from build123d import *

# Parameters (mm, degrees)
F0_R     = 5
F0_W     = 15
F0_H     = 20
F1_DEPTH = 1.6
F2_R     = 1
F3_DEPTH = 25


with BuildPart() as f1:
    # F0 (on Front) → F1 (new body)
    with BuildSketch(Plane.XZ):
        Polygon((28, 71), (-24.5, 71), (-24.5, 30), (-28, 30), (-28, -102), (8, -102), (8, -82), (28, -82), align=None)
        with Locations((-14.37, -78.52)):
            Circle(F0_R, mode=Mode.SUBTRACT)
        with Locations((-14.37, -55.02)):
            Circle(F0_R, mode=Mode.SUBTRACT)
        with Locations((-14.58, -35.06)):
            Rectangle(F0_W, F0_H, mode=Mode.SUBTRACT)
        Polygon((1.52, -25.06), (9.02, -25.06), (16.52, -25.06), (16.52, -45.06), (9.02, -45.06), (1.52, -45.06), align=None, mode=Mode.SUBTRACT)
    extrude(amount=-F1_DEPTH)

    # F2 (on face) → F3 (cut)
    with BuildSketch(Plane.XZ):
        with Locations((0, 25.5)):
            Circle(F2_R)
        with Locations((0, 68)):
            Circle(F2_R)
        with Locations((23, 17)):
            Circle(F2_R)
        with Locations((23, -17)):
            Circle(F2_R)
        with Locations((-23, -10)):
            Circle(F2_R)
        with Locations((0, -58)):
            Circle(F2_R)
        with Locations((-5, -78.5)):
            Circle(F2_R)
    extrude(amount=-F3_DEPTH, mode=Mode.SUBTRACT)


solid = f1.part
Could you check a few things on this model? Use its own coordinates, in mm. Give positions to 0.01 mm unless a question says otherwise; leave off trailing zeros. Order: outer loops, then holes, each group sorted by start corner. A loop starts at its lowest first (then second) coordinate and runs counter-clockwise, first axis right, second up.
Item 1: If we section it at B-B, the plane y = 0.8: Count the separate pieces of the cut face and the enclosed holes in it, plus the area to 3 significant figures.
Item 2: If we section it at C-C, the plane z = 54: Write out the boundary of the cut face in (x, y), plus the area to 3 significant figures.
Item 3: I'm going to push flat-ended pins straight in: pin 1 (0.5 mm diameter, centred on y = 1, z = 56.5, fed in from -X); pin 2 (1.8 mm diameter, centred on x = -5, z = -78.5, fed in from +Y); pin 3 (13 mm diameter, centred on x = -14.37, z = -78.52, fed in from -Y). Where does each tip first touch, or does it pass through?
Item 4: If we mould it in two halves opening along X, with no side actions, what happens to faces 1 (the face through (0, 0, -14)), 2 (the face through (-9.6, 0.79, -53.52))? For each: pulls with the +X half, pulls with the -X half, needs draft (parallel to the pull), parting line crosses it, or undercut.
Item 5: If we section it at A-A, the plane x = -12: Write out the boundary of the cut face in (y, z), plus the area to 3 significant figures.
Item 6: I need wall thicknesses on line 1 (Z direction, x = 0, y = 1); line 2 (X direction, y = 1.3, z = -43.5); line 3 (X direction, y = 0.6, z = -78.5). Which ranges of each line are inside material? Lowest first, please.
Values:
1. separate pieces: 1
1. enclosed holes: 11
1. area: 8,370 mm2
2. outline: (-24.5, 0) - (28, 0) - (28, 1.6) - (-24.5, 1.6) - close
2. area: 84.0 mm2
3. pin 1: stops at x = -24.5
3. pin 2: passes through
3. pin 3: stops at y = 0
4. face 1: needs draft
4. face 2: undercut
5. outline: (0, -102) - (1.6, -102) - (1.6, -82.92) - (0, -82.92) - close; (0, -74.12) - (1.6, -74.12) - (1.6, -59.42) - (0, -59.42) - close; (0, -50.62) - (1.6, -50.62) - (1.6, -45.06) - (0, -45.06) - close; (0, -25.06) - (1.6, -25.06) - (1.6, 71) - (0, 71) - close
5. area: 217 mm2
6. line 1: z = -102 to -59, -57 to 24.5, 26.5 to 67, 69 to 71
6. line 2: x = -28 to -22.08, -7.08 to 1.52, 16.52 to 28
6. line 3: x = -28 to -19.37, -9.37 to -6, -4 to 28
